```python
from build123d import *

# Parameters (mm, degrees)
SKETCH1_W           = 3.4
SKETCH1_H           = 24
BOSS_EXTRUDE1_DEPTH = 0.3
CUT_EXTRUDE1_DEPTH  = 1.3
CUT_EXTRUDE2_DEPTH  = 1.3
LPATTERN1_COUNT     = 9
LPATTERN1_PITCH     = 1.25
CUT_EXTRUDE4_DEPTH  = 1.3


with BuildPart() as part:
    # Sketch1 → Boss-Extrude1 (new body)
    with BuildSketch(Plane.XY):
        Rectangle(SKETCH1_W, SKETCH1_H)
    extrude(amount=-BOSS_EXTRUDE1_DEPTH)

    # Sketch2 → Cut-Extrude1 (cut, through all)
    with BuildSketch(Plane.XY):
        with BuildLine():
            Line((-1.7, -12), (-0.7, -12))
            Line((-0.7, -12), (-0.7, 0))
            ThreePointArc((-0.7, 0), (-0.763092877, 0.185865622), (-0.926295644, 0.294914224))
            Line((-0.926295644, 0.294914224), (-1.581411047, 0.470451868))
            ThreePointArc((-1.581411047, 0.470451868), (-1.666936534, 0.527598171), (-1.7, 0.625))
            Line((-1.7, 0.625), (-1.7, -12))
        make_face()
    extrude(amount=-CUT_EXTRUDE1_DEPTH, mode=Mode.SUBTRACT)

    # Sketch3 → Cut-Extrude2 (cut, through all)
    with BuildSketch(Plane.XY):
        with BuildLine():
            Line((-1.581411047, 0.779548132), (-0.926295644, 0.955085776))
            ThreePointArc((-0.926295644, 0.955085776), (-0.7, 1.25), (-0.926295644, 1.544914224))
            Line((-0.926295644, 1.544914224), (-1.581411047, 1.720451868))
            ThreePointArc((-1.581411047, 1.720451868), (-1.666936534, 1.777598171), (-1.7, 1.875))
            Line((-1.7, 1.875), (-1.7, 0.625))
            ThreePointArc((-1.7, 0.625), (-1.666936534, 0.722401829), (-1.581411047, 0.779548132))
        make_face()
    cut_extrude2 = extrude(amount=-CUT_EXTRUDE2_DEPTH, mode=Mode.SUBTRACT)

    # LPattern1: Cut-Extrude2 ×9
    with Locations(*[(0, i * LPATTERN1_PITCH, 0) for i in range(1, LPATTERN1_COUNT)]):
        add(cut_extrude2, mode=Mode.SUBTRACT)

    # Sketch4 → Cut-Extrude4 (cut, through all)
    with BuildSketch(Plane.XY):
        with BuildLine():
            Line((-0.7, 11.25), (-0.7, 12))
            Line((-0.7, 12), (-1.7, 12))
            Line((-1.7, 12), (-1.7, 11.875))
            ThreePointArc((-1.7, 11.875), (-1.666936534, 11.777598171), (-1.581411047, 11.720451868))
            Line((-1.581411047, 11.720451868), (-0.926295644, 11.544914224))
            ThreePointArc((-0.926295644, 11.544914224), (-0.763092877, 11.435865622), (-0.7, 11.25))
        make_face()
    extrude(amount=-CUT_EXTRUDE4_DEPTH, mode=Mode.SUBTRACT)


solid = part.part
```
Geometry check sheet. Reference: the model listing, model coordinates, mm. Give positions to 0.01 mm unless a question says otherwise; leave off trailing zeros. Order: outer loops, then holes, each group sorted by start corner. A loop starts at its lowest first (then second) coordinate and runs counter-clockwise, first axis right, second up. Notation, with made-up numbers: (26.25, 71) - (60.25, 71) arc R21 ccw to (60.25, 77) - close; hole circle Ø3 at (88.25, 20.25). An arc over 180 degrees is marked (long way). Write item = value, one per line. Start each with the question number.
1) Section check B-B (x = -1.35). Count the separate pieces of the cut face and the enclosed holes in it, then the cut area to 3 significant figures.
2) Section check A-A (y = -4.25). Enter the section's corners in (x, z).
3) Scan lines: L1, parallel to X at y = -9.5, z = -0.05; L2, parallel to X at y = 6, z = -0.15. Record each from-to range of solid material in increasing order.
Geometry check:
q1.separate_pieces = 9
q1.enclosed_holes = 0
q1.area = 1.17 mm2
q2.outline = (-0.7, -0.3) - (1.7, -0.3) - (1.7, 0) - (-0.7, 0) - close
q3.L1 = -0.7 to 1.7
q3.L2 = -0.83 to 1.7
